from build123d import *

# Parameters (mm, degrees)
SKETCH_1_R      = 22.5
EXTRUDE_1_DEPTH = 3
SKETCH_2_R      = 1.4
EXTRUDE_2_DEPTH = 3


with BuildPart() as part:
    # Эскиз1 → Вытянуть1 (new body)
    with BuildSketch(Plane(origin=(0, 0, 0), x_dir=(1, 0, 0), z_dir=(0, 1, 0))):
        with Locations(Location((0, 0, 0), (0, 0, 270))):
            Circle(SKETCH_1_R)
        with BuildLine():
            Line((1.9, 3.689512163), (-1.9, 3.689512163))
            ThreePointArc((-1.9, 3.689512163), (-2.934493142, -2.934493142), (3.689512163, -1.9))
            Line((3.689512163, -1.9), (3.689512163, 1.9))
            ThreePointArc((3.689512163, 1.9), (2.934493142, 2.934493142), (1.9, 3.689512163))
        make_face(mode=Mode.SUBTRACT)
    extrude(amount=EXTRUDE_1_DEPTH)

    # Эскиз2 → Вытянуть2 (add)
    with BuildSketch(Plane.XZ):
        with Locations(Location((0, 12.5, 0), (0, 0, 90))):
            Circle(SKETCH_2_R)
        with Locations(Location((0, -12.5, 0), (0, 0, 90))):
            Circle(SKETCH_2_R)
    extrude(amount=EXTRUDE_2_DEPTH)


solid = part.part
Verification items for the finished model (mm, model axes). A direction names the side the tool comes from. Coordinates: 2 decimals unless noted, no trailing zeros. Order: outer loops, then holes, each group sorted by start corner. A loop starts at its lowest first (then second) coordinate and runs counter-clockwise, first axis right, second up. Notation, with made-up numbers: (12, 29.5) -> (44, 29.5) arc R9 ccw to (44, 45.5) -> close; hole circle Ø4 at (70, 12.5). An arc over 180 degrees is marked (long way). Use CSV: the item, a comma, the result in double quotes. Start each with the question number.
Q1. Draft check along X on faces 4 (the flat face through (-5, 3, 0)), 5 (the cylindrical face through (-0.06, -1.48, -13.9)), 6 (the flat face through (0, 1, -3.69)). Enter one of: +X half, -X half, draft (parallel to the pull), parting line (faces both ways), or undercut.
Q2. Section check C-C, the plane y = -2.4. Record the cut outline in (x, z).
Q3. Section check D-D, the plane z = 13. Record the cut outline in (x, y), and give its area (3 significant figures).
Q4. Section check B-B, the plane x = 0. Record the cut outline in (y, z), and give its area (3 significant figures).
Q5. Depth check by flat-ended pin: P1, Ø6, axis at x = -6, z = -13, coming from the -Y side; P2, Ø2, axis at y = -1.5, z = 10.5, coming from the +X side; P3, Ø0.9, axis at x = 1, y = 1.5, coming from the +Z side. Enter the tip coordinate at first touch or a pass-through.
Q6. Tool access check on faces 1 (the cylindrical face through (-0.06, -1.48, 11.1)), 2 (the cylindrical face through (2.95, 1.48, -2.92)), 3 (the flat face through (0, -3, -13)). Record the directions out of +Z, -Z, +X, -X, +Y, -Y that give a thin tool (end or side, any length) a straight path to the whole face; none if there is none.
Q7. Thickness scan on line 1 along X through (y, z) = (1.5, 0); line 2 along Y through (x, z) = (1.5, -8); line 3 along Z through (x, y) = (3, 0.95). Record the ranges inside material, lowest first.
Q8. Section check A-A, the plane z = 0. Record the cut outline in (x, y), and give its area (3 significant figures).
Returned:
1,face 4,"draft"
1,face 5,"parting line"
1,face 6,"undercut"
2,outline,"circle Ø2.8 at (0, -12.5); circle Ø2.8 at (0, 12.5)"
3,outline,"(-18.36, 0) -> (-1.31, 0) -> (-1.31, -3) -> (1.31, -3) -> (1.31, 0) -> (18.36, 0) -> (18.36, 3) -> (-18.36, 3) -> close"
3,area,"118 mm^2"
4,outline,"(-3, -13.9) -> (0, -13.9) -> (0, -22.5) -> (3, -22.5) -> (3, -3.69) -> (0, -3.69) -> (0, -11.1) -> (-3, -11.1) -> close; (-3, 11.1) -> (0, 11.1) -> (0, 4.15) -> (3, 4.15) -> (3, 22.5) -> (0, 22.5) -> (0, 13.9) -> (-3, 13.9) -> close"
4,area,"128 mm^2"
5,P1,"stops at y = 0"
5,P2,"stops at x = 0.98"
5,P3,"stops at z = 22.49"
6,face 1,"-Y"
6,face 2,"+Y, -Y"
6,face 3,"+Z, -Z, +X, -X, -Y"
7,line 1,"x = -22.5 to -4.15, 3.69 to 22.5"
7,line 2,"y = 0 to 3"
7,line 3,"z = -22.3 to -2.87, 2.87 to 22.3"
8,outline,"(-22.5, 0) -> (-4.15, 0) -> (-4.15, 3) -> (-22.5, 3) -> close; (3.69, 0) -> (22.5, 0) -> (22.5, 3) -> (3.69, 3) -> close"
8,area,"111 mm^2"
